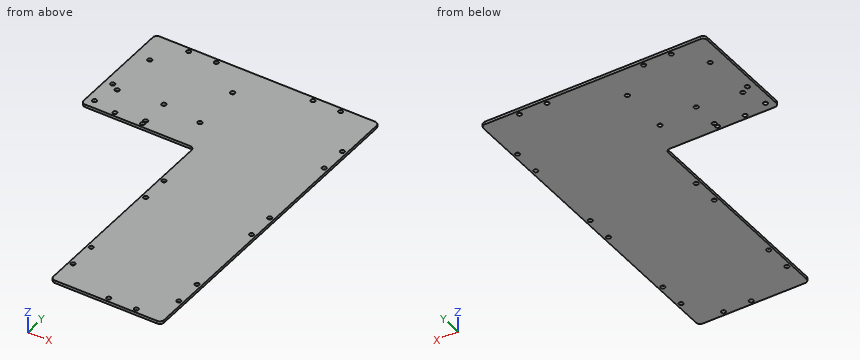
```python
from build123d import *

# Parameters (mm, degrees)
SKETCH_1_W          = 82
SKETCH_1_H          = 82
EXTRUDE_1_DEPTH     = 2
SKETCH_2_R          = 1.55
SKETCH_2_R_2        = 1.6
CUT_EXTRUDE_1_DEPTH = 233.907707043
FILLET_1_R          = 3
SKETCH_4_R          = 1.6
CUT_EXTRUDE_2_DEPTH = 233.907707043


with BuildPart() as part:
    # 草图1 → 凸台-拉伸1 (new body)
    with BuildSketch(Plane.XY):
        Rectangle(SKETCH_1_W, SKETCH_1_H)
        Polygon((121, 41), (41, 41), (41, -41), (41, -199), (121, -199), align=None)
    extrude(amount=EXTRUDE_1_DEPTH)

    # 草图2 → 切除-拉伸1 (cut, through all)
    with BuildSketch(Plane.XY.offset(2)):
        with Locations((-15, 38)):
            Circle(SKETCH_2_R)
        with Locations((5, 38)):
            Circle(SKETCH_2_R)
        with Locations((-18.5, -38)):
            Circle(SKETCH_2_R)
        with Locations((1.5, -38)):
            Circle(SKETCH_2_R)
        with Locations((-30, 18)):
            Circle(SKETCH_2_R_2)
        with Locations((30, 18)):
            Circle(SKETCH_2_R_2)
        with Locations((30, -18)):
            Circle(SKETCH_2_R_2)
        with Locations((-30, -18)):
            Circle(SKETCH_2_R_2)
        with Locations((44, -179)):
            Circle(SKETCH_2_R)
        with Locations((44, -159)):
            Circle(SKETCH_2_R)
        with Locations((101, -196)):
            Circle(SKETCH_2_R)
        with Locations((81, -196)):
            Circle(SKETCH_2_R)
        with Locations((44, -99)):
            Circle(SKETCH_2_R)
        with Locations((44, -79)):
            Circle(SKETCH_2_R)
        with Locations((118, 5)):
            Circle(SKETCH_2_R)
        with Locations((118, -15)):
            Circle(SKETCH_2_R)
        with Locations((118, -75)):
            Circle(SKETCH_2_R)
        with Locations((118, -95)):
            Circle(SKETCH_2_R)
        with Locations((118, -175)):
            Circle(SKETCH_2_R)
        with Locations((118, -155)):
            Circle(SKETCH_2_R)
        with Locations((95, 38)):
            Circle(SKETCH_2_R)
        with Locations((75, 38)):
            Circle(SKETCH_2_R)
    extrude(amount=-CUT_EXTRUDE_1_DEPTH, mode=Mode.SUBTRACT)

    # 圆角1
    fillet_1_edges = [part.edges().sort_by_distance(p)[0] for p in [
        (-41, -41, 1),
        (-41, 41, 1),
        (121, 41, 1),
        (121, -199, 1),
        (41, -199, 1),
        (41, -41, 1),
    ]]
    fillet(fillet_1_edges, radius=FILLET_1_R)

    # 草图4 → 切除-拉伸2 (cut, through all)
    with BuildSketch(Plane.XY.offset(2)):
        with Locations((-35.434500029, -34.624495654)):
            Circle(SKETCH_4_R)
        with Locations((1.595499971, -34.624495654)):
            Circle(SKETCH_4_R)
        with Locations((1.595499971, -14.624495654)):
            Circle(SKETCH_4_R)
        with Locations((-35.434500029, -14.624495654)):
            Circle(SKETCH_4_R)
    extrude(amount=-CUT_EXTRUDE_2_DEPTH, mode=Mode.SUBTRACT)


solid = part.part
```
Design review of the part built by this model. Coordinates are the model's own, in mm. Round coordinates to 2 decimals unless told otherwise and drop trailing zeros. Write each loop counter-clockwise with the first axis right and the second up, starting at its lowest first coordinate (ties: lowest second). Pieces come first, ordered by that corner, then holes.
Item 1: For probe 1 along Y at (x, z) = (44, 0.4); probe 2 along Y at (x, z) = (-30, 0.55); probe 3 along Y at (x, z) = (45, 0.25), list the stretches that pass through material, from the lowest coordinate up.
Item 2: We need section B-B on z = 1.4. State how many separate pieces and enclosed holes the cut face has, and give its area (3 significant figures).
Item 3: Clearance check with flat-ended pins moving along their axes: pin 1 Ø5 at (x, y) = (95, 38) entering from -Z; pin 2 Ø2.5 at (x, y) = (118, -15) entering from -Z; pin 3 Ø1 at (x, z) = (-10, 0.5) entering from -Y. State where each tip first meets the part, or that it passes through.
Item 4: We need section A-A on y = -123. Write out the cut boundary in (x, z).
Returned:
1. probe 1: y = -199 to -180.55, -177.45 to -160.55, -157.45 to -100.55, -97.45 to -80.55, -77.45 to 41
1. probe 2: y = -41 to -19.6, -16.4 to 16.4, 19.6 to 41
1. probe 3: y = -199 to -180.18, -177.82 to -160.18, -157.82 to -100.18, -97.82 to -80.18, -77.82 to 41
2. separate pieces: 1
2. enclosed holes: 26
2. area: 25,700 mm2
3. pin 1: stops at z = 0
3. pin 2: passes through
3. pin 3: stops at y = -41
4. outline: (41, 0) - (121, 0) - (121, 2) - (41, 2) - close
